Drawing for the job (mm, zero at the part's lowest x, y, z). A direction names the side the tool comes from. Give positions to 0.01 mm unless a question says otherwise; leave off trailing zeros. Write each loop counter-clockwise with the first axis right and the second up, starting at its lowest first coordinate (ties: lowest second). Pieces come first, ordered by that corner, then holes. Notation, with made-up numbers: M 39,-21 L 60,-21 A27 cw 60,11 Z; hole C 86,30 d7. An arc over 180 degrees is marked long. Use CSV: the item, a comma, the result in double quotes. Start each with the question number.
1. Band-saw the part on A-A, the plane x = 2. List the corners of the cut face in (y, z), then the cut area to 3 significant figures.
2. Band-saw the part on C-C, the plane y = 4.5. List the corners of the cut face in (x, z), then the cut area to 3 significant figures.
3. Drop flat-ended pins along their axis: pin 1 Ø4 at (y, z) = (8, 5) entering from -X; pin 2 Ø2.5 at (y, z) = (6, 6) entering from +X; pin 3 Ø1.8 at (x, y) = (24, 2) entering from +Z; pin 4 Ø2 at (x, y) = (23.5, 2.5) entering from -Z. Give the stop position or say it passes through.
4. Band-saw the part on D-D, the plane y = 1.75. List the corners of the cut face in (x, z), then the cut area to 3 significant figures.
5. Mould opens along X. For the marked faces 1, 2 and 3 say: pulls with the +X half, pulls with the -X half, needs draft (parallel to the pull), parting line crosses it, or undercut.
6. Drill centre lines: line 1 along Y through (x, z) = (2, 10.7); line 2 along X through (y, z) = (5.75, 7.5); line 3 along Z through (x, y) = (13, 6.75). Where is each one in solid material? Low to high. Write a range as from..to.
7. 3-axis set-ups, long thin cutter, end or side, ignore diameter. For the marked faces 4, 5 and 6: which of +Z, -Z, +X, -X, +Y, -Y reach the whole face in a straight line?
8. Band-saw the part on B-B, the plane z = 6. List the corners of the cut face in (x, y), then the cut area to 3 significant figures.
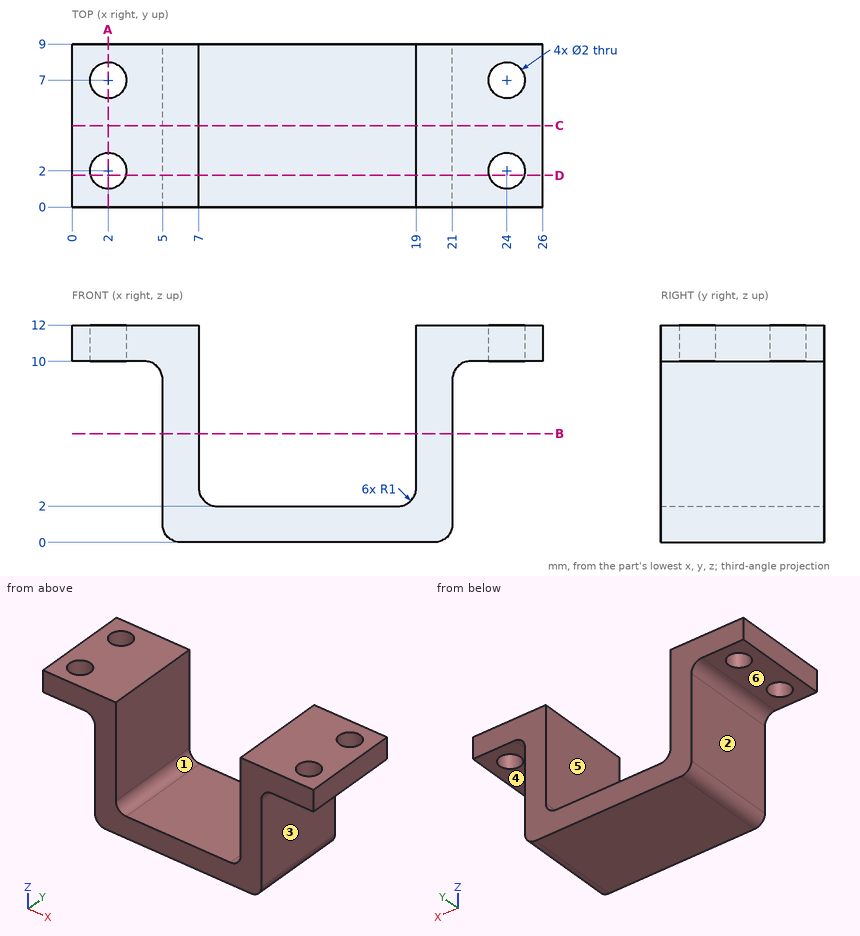
Output:
1,outline,"M 0,10 L 1,10 L 1,12 L 0,12 Z; M 3,10 L 6,10 L 6,12 L 3,12 Z; M 8,10 L 9,10 L 9,12 L 8,12 Z"
1,area,"10.0 mm²"
2,outline,"M 0,10 L 4,10 A1 cw 5,9 L 5,1 A1 ccw 6,0 L 20,0 A1 ccw 21,1 L 21,9 A1 cw 22,10 L 26,10 L 26,12 L 19,12 L 19,3 A1 cw 18,2 L 8,2 A1 cw 7,3 L 7,12 L 0,12 Z"
2,area,"92.4 mm²"
3,pin 1,"stops at x = 5"
3,pin 2,"stops at x = 21"
3,pin 3,"passes through"
3,pin 4,"stops at z = 10"
4,outline,"M 0,10 L 1.03,10 L 1.03,12 L 0,12 Z; M 2.97,10 L 4,10 A1 cw 5,9 L 5,1 A1 ccw 6,0 L 20,0 A1 ccw 21,1 L 21,9 A1 cw 22,10 L 23.03,10 L 23.03,12 L 19,12 L 19,3 A1 cw 18,2 L 8,2 A1 cw 7,3 L 7,12 L 2.97,12 Z; M 24.97,10 L 26,10 L 26,12 L 24.97,12 Z"
4,area,"84.7 mm²"
5,face 1,"undercut"
5,face 2,"pulls with the -X half"
5,face 3,"pulls with the +X half"
6,line 1,"y = 0..1, 3..6, 8..9"
6,line 2,"x = 5..7, 19..21"
6,line 3,"z = 0..2"
7,face 4,"-Z, +X, +Y, -Y"
7,face 5,"+Z, +Y, -Y"
7,face 6,"-Z, -X, +Y, -Y"
8,outline,"M 5,0 L 7,0 L 7,9 L 5,9 Z; M 19,0 L 21,0 L 21,9 L 19,9 Z"
8,area,"36.0 mm²"
